Could you check a few things on this model? Use its own coordinates, in mm. Give positions to 0.01 mm unless a question says otherwise; leave off trailing zeros. Write each loop counter-clockwise with the first axis right and the second up, starting at its lowest first coordinate (ties: lowest second). Pieces come first, ordered by that corner, then holes. Notation, with made-up numbers: M -31,48.25 L 16,48.25 A15 ccw 16,67.25 Z; hole C 66.5,6.25 d9. An arc over 180 degrees is marked long. Write each question's results on one line, items separated by ' | '. Start each with the question number.
from build123d import *

# Parameters (mm, degrees)
F1_ANGLE = 180
F2_R     = 5.08


with BuildPart() as f1:
    # F0 (on Front) → F1 (revolve)
    with BuildSketch(Plane.XZ):
        Polygon((-45.289915, 0), (-9.171271, 0), (-9.171271, 6.151464), (-19.96652, 13.392183), (-9.171271, 21.291147), (-9.171271, 28.001834), (-45.289915, 28.001834), align=None)
    revolve(axis=Axis((0, 0, 31.041022), (0, 0, 1)), revolution_arc=F1_ANGLE)

    # F2
    f2_edges = [f1.edges().sort_by_distance(p)[0] for p in [
        (0, -45.289915, 0),
    ]]
    fillet(f2_edges, radius=F2_R)


solid = f1.part
Q1. Please list where these lines run through material, in increasing order: line 1 (X direction, y = -7.5, z = 20.5); line 2 (X direction, y = -8, z = 18.25); line 3 (X direction, y = -35, z = 3.5). Write a range as [from, to].
Q2. If we mould it in two halves opening along X, with no side actions, what happens to faces 1 (the face through (-1, -18, 28.002)), 2 (the face through (-0.243, -11.043, 7.409)), 3 (the face through (-1, -45.28, 16.38))? For each: pulls with the +X half, pulls with the -X half, needs draft (parallel to the pull), parting line crosses it, or undercut.
Q3. If we section it at A-A (x = 0): Please give me the cut outline in (y, z).
Q4. I'm going to push flat-ended pins straight in: P1, Ø6, axis at x = -31.5, y = -35.5, coming from the -Z side; P2, Ø1.5, axis at y = -29, z = 11.5, coming from the +X side; P3, Ø10, axis at y = -37, z = 3, coming from the +X side. Where does each tip first touch, or does it pass through?
Q5. If we section it at B-B (z = 24.5): Please give me the cut outline in (x, y).
Q6. If we section it at C-C (z = 18.25): Please give me the cut outline in (x, y) (1 decimal), plus the area to 3 significant figures.
Determined:
1) line 1: x = [-44.66, -6.99], [6.99, 44.66] | line 2: x = [-44.58, -10.66], [10.66, 44.58] | line 3: x = [-28.34, 28.34]
2) face 1: needs draft | face 2: undercut | face 3: parting line crosses it
3) outline: M -45.29,5.08 A5.08 ccw -40.21,0 L -9.17,0 L -9.17,6.15 L -19.97,13.39 L -9.17,21.29 L -9.17,28 L -45.29,28 Z
4) P1: stops at z = 2.3 | P2: stops at x = 35.4 | P3: stops at x = 31.79
5) outline: M -45.29,0 A45.29 ccw 45.29,0 L 9.17,0 A9.17 cw -9.17,0 Z
6) outline: M -45.3,0 A45.3 ccw 45.3,0 L 13.3,0 A13.3 cw -13.3,0 Z | area: 2,940 mm²
